CAD build for the part. Positions are in the model's coordinates, mm. Face numbers are marked on the shaded views. A direction names the side the tool comes from. Give positions to 0.01 mm unless a question says otherwise; leave off trailing zeros. Order: outer loops, then holes, each group sorted by start corner. A loop starts at its lowest first (then second) coordinate and runs counter-clockwise, first axis right, second up.
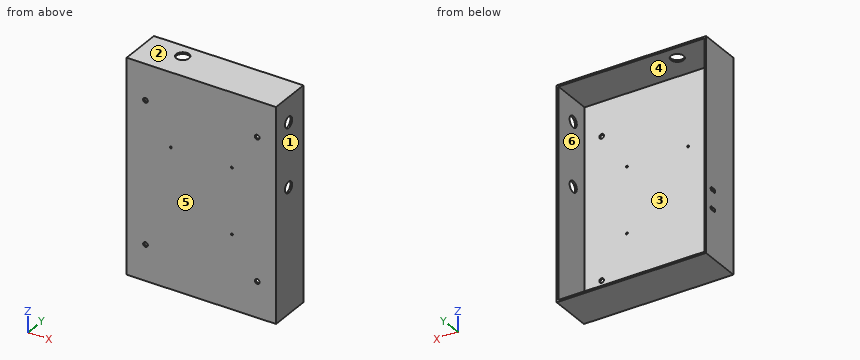
from build123d import *

# Parameters (mm, degrees)
SKETCH1_W             = 254
SKETCH1_H             = 361
SKETCH1_W_2           = 248
SKETCH1_H_2           = 355
BOSS_EXTRUDE1_DEPTH   = 3
BOSS_EXTRUDE2_START   = 3
SKETCH1_3_W           = 254
SKETCH1_3_H           = 361
SKETCH1_3_W_2         = 248
SKETCH1_3_H_2         = 355
BOSS_EXTRUDE2_DEPTH   = 69
SKETCH2_R             = 9.5
CUT_EXTRUDE1_DEPTH    = 3
SKETCH3_R             = 11
CUT_EXTRUDE2_DEPTH    = 3
SKETCH4_R             = 3.25
CUT_EXTRUDE3_DEPTH    = 3
SKETCH5_R             = 4
CUT_EXTRUDE4_DEPTH    = 3
M4X0_7_TAPPED_HOLE1_D = 3.3


with BuildPart() as part:
    # Sketch1 → Boss-Extrude1 (new body)
    # profile 1 of 2: a face of its own
    with BuildSketch(Plane(origin=(0, 0, 0), x_dir=(1, 0, 0), z_dir=(0, 1, 0))):
        with Locations((124, -177.5)):
            Rectangle(SKETCH1_W, SKETCH1_H)
        with Locations((124, -177.5)):
            Rectangle(SKETCH1_W_2, SKETCH1_H_2, mode=Mode.SUBTRACT)
    # profile 2 of 2: a face of its own
    with BuildSketch(Plane(origin=(0, 0, 0), x_dir=(1, 0, 0), z_dir=(0, 1, 0))):
        with Locations((124, -177.5)):
            Rectangle(SKETCH1_W_2, SKETCH1_H_2)
    extrude(amount=BOSS_EXTRUDE1_DEPTH)

    # Sketch1<3> → Boss-Extrude2 (add)
    with BuildSketch(Plane(origin=(0, 0, 0), x_dir=(1, 0, 0), z_dir=(0, 1, 0)).offset(BOSS_EXTRUDE2_START)):
        with Locations((124, -177.5)):
            Rectangle(SKETCH1_3_W, SKETCH1_3_H)
        with Locations((124, -177.5)):
            Rectangle(SKETCH1_3_W_2, SKETCH1_3_H_2, mode=Mode.SUBTRACT)
    extrude(amount=BOSS_EXTRUDE2_DEPTH)

    # Sketch2 → Cut-Extrude1 (cut)
    with BuildSketch(Plane(origin=(251, 0, 0), x_dir=(0, 0, -1), z_dir=(1, 0, 0))):
        with Locations((-316, 33)):
            Circle(SKETCH2_R)
        with Locations((-208, 33)):
            Circle(SKETCH2_R)
    extrude(amount=-CUT_EXTRUDE1_DEPTH, mode=Mode.SUBTRACT)

    # Sketch3 → Cut-Extrude2 (cut)
    with BuildSketch(Plane.XY.offset(358)):
        with Locations((62, 47)):
            Circle(SKETCH3_R)
    extrude(amount=-CUT_EXTRUDE2_DEPTH, mode=Mode.SUBTRACT)

    # Sketch4 → Cut-Extrude3 (cut)
    with BuildSketch(Plane.ZY.offset(3)):
        with Locations((79, 51.25)):
            Circle(SKETCH4_R)
        with Locations((79, 56.75)):
            Circle(SKETCH4_R)
        with Locations((111, 56.75)):
            Circle(SKETCH4_R)
        with Locations((111, 51.25)):
            Circle(SKETCH4_R)
    extrude(amount=-CUT_EXTRUDE3_DEPTH, mode=Mode.SUBTRACT)

    # Sketch5 → Cut-Extrude4 (cut)
    with BuildSketch(Plane(origin=(0, 3, 0), x_dir=(1, 0, 0), z_dir=(0, 1, 0))):
        with Locations(Location((29, -297.5, 0), (0, 0, 270))):
            Circle(SKETCH5_R)
        with Locations(Location((219, -297.5, 0), (0, 0, 270))):
            Circle(SKETCH5_R)
        with Locations(Location((29, -57.5, 0), (0, 0, 270))):
            Circle(SKETCH5_R)
        with Locations(Location((219, -57.5, 0), (0, 0, 270))):
            Circle(SKETCH5_R)
    extrude(amount=-CUT_EXTRUDE4_DEPTH, mode=Mode.SUBTRACT)

    # M4x0.7 Tapped Hole1 (through all)
    with Locations(Plane(origin=(0, 3, 0), x_dir=(1, 0, 0), z_dir=(0, 1, 0))):
        with Locations((72, -233), (176, -233), (176, -122)):
            Hole(M4X0_7_TAPPED_HOLE1_D / 2)


solid = part.part
1. Wall check: line 1 (X direction, y = 2.4, z = 233); line 2 (X direction, y = 1, z = 297); line 3 (X direction, y = 26, z = 307.5). Give the ranges that are in metal, low to high.
2. Saw through at B-B on y = 17. Give the cut face in (x, z), plus the area to 3 significant figures.
3. Mould opens along X. For the marked faces 1, 2, 3 and 4 say: released by +X, released by -X, zero draft, split by the parting line, or undercut.
4. 3-axis set-ups, long thin cutter, end or side, ignore diameter. For the marked faces 5 and 6: which of +Z, -Z, +X, -X, +Y, -Y reach the whole face in a straight line?
5. Saw through at D-D on z = 310.5. Give the cut face in (x, y).
6. Pin check, flat tips, straight feed: P1, Ø4, axis at y = 56.75, z = 79, coming from the -X side; P2, Ø4, axis at x = 176, z = 122, coming from the +Y side. Stop position of each tip, or through.
7. Saw through at A-A on x = 29. Give the cut face in (y, z), plus the area to 3 significant figures.
8. Saw through at C-C on z = 26. Give the cut face in (x, y).
Reported:
1. line 1: x = -3 to 70.35, 73.65 to 174.35, 177.65 to 251
1. line 2: x = -3 to 25.03, 32.97 to 215.03, 222.97 to 251
1. line 3: x = -3 to 0, 248 to 251
2. outline: (-3, -3) - (251, -3) - (251, 358) - (-3, 358) - close; hole (0, 0) - (248, 0) - (248, 355) - (0, 355) - close
2. area: 3,650 mm2
3. face 1: released by +X
3. face 2: zero draft
3. face 3: undercut
3. face 4: undercut
4. face 5: +Z, -Z, +X, -X, -Y
4. face 6: +Y
5. outline: (-3, 0) - (251, 0) - (251, 25.25) - (248, 25.25) - (248, 3) - (0, 3) - (0, 72) - (-3, 72) - close; (248, 40.75) - (251, 40.75) - (251, 72) - (248, 72) - close
6. P1: stops at x = 248
6. P2: stops at y = 3
7. outline: (0, -3) - (72, -3) - (72, 0) - (3, 0) - (3, 53.5) - (0, 53.5) - close; (0, 61.5) - (3, 61.5) - (3, 293.5) - (0, 293.5) - close; (0, 301.5) - (3, 301.5) - (3, 355) - (72, 355) - (72, 358) - (0, 358) - close
7. area: 1,450 mm2
8. outline: (-3, 0) - (251, 0) - (251, 72) - (248, 72) - (248, 3) - (0, 3) - (0, 72) - (-3, 72) - close
